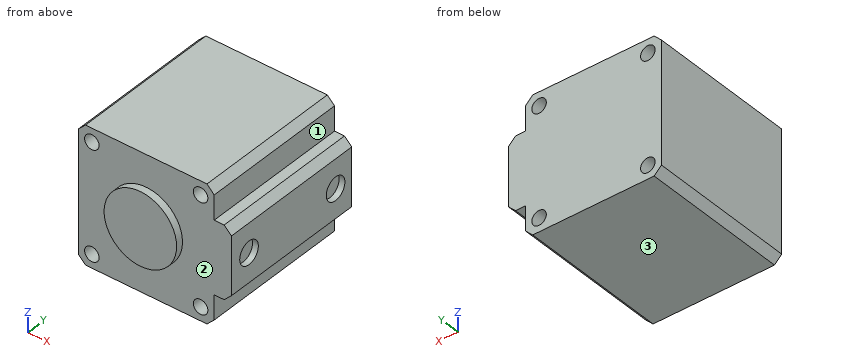
Autodesk Inventor part; units mm, degrees
ref_plane "YZ Plane" through (0, 0, 0) normal (1, 0, 0) x (0, 1, 0)
ref_plane "XZ Plane" through (0, 0, 0) normal (0, 1, 0) x (-1, 0, 0)
ref_plane "XY Plane" through (0, 0, 0) normal (0, 0, 1) x (1, 0, 0)
sketch "Sketch1" plane through (0, 0, 0) normal (0, 1, 0) x (-1, 0, 0)
  line L0 (0, 0) -> (75, 0)
  line L1 (75, 0) -> (75, -75)
  line L2 (75, -75) -> (0, -75)
  line L3 (0, -75) -> (0, 0)
  dimension "d0" = 75
  dimension "d1" = 75
extrude "Extrusion1" add sketch "Sketch1" along normal blind 82
sketch "Sketch2" plane through (0, 0, 0) normal (0, -1, 0) x (1, 0, 0)
  circle A0 centre (-37.5, -37.5) radius 20
  line L0 (0, -75) -> (0, 0)
  line L1 (-75, -75) -> (0, -75)
  dimension "d4" = 40
  dimension "d5" = 37.5
  dimension "d6" = 37.5
extrude "Extrusion2" add sketch "Sketch2" along normal blind 4
sketch "Sketch4" plane through (0, 0, 0) normal (0, -1, 0) x (1, 0, 0)
  circle A0 centre (-67.5, -7.5) radius 4
  circle A1 centre (-7.5, -7.5) radius 4
  circle A2 centre (-7.5, -67.5) radius 4
  circle A3 centre (-67.5, -67.5) radius 4
  line L0 (0, 0) -> (-75, 0)
  line L1 (0, -75) -> (0, 0)
  dimension "d12" = 8
  dimension "d13" = 8
  dimension "d14" = 8
  dimension "d15" = 8
  dimension "d16" = 60
  dimension "d17" = 60
  dimension "d18" = 60
  dimension "d19" = 60
  dimension "d20" = 60
  dimension "d21" = 60
  dimension "d22" = 7.5
  dimension "d23" = 7.5
extrude "Extrusion4" cut sketch "Sketch4" against normal blind 120.8875
sketch "Sketch5" plane through (0, 0, 0) normal (1, 0, 0) x (0, 0, -1)
  line L0 (75, 0) -> (0, 0)
  line L1 (75, 82) -> (0, 82)
  line L2 (17.5, 0) -> (57.5, 0)
  line L3 (57.5, 0) -> (57.5, 82)
  line L4 (57.5, 82) -> (17.5, 82)
  line L5 (17.5, 82) -> (17.5, 0)
  line L6 (0, 0) -> (0, 82)
  dimension "d26" = 40
  dimension "d27" = 17.5
extrude "Extrusion5" add sketch "Sketch5" along normal blind 9.5 contours L0 L5 L1 L3
sketch "Sketch6" plane through (9.5, 0, 0) normal (1, 0, 0) x (0, 0, -1)
  circle A0 centre (37.5, 12) radius 6.35
  circle A1 centre (37.5, 71) radius 6.35
  line L0 (57.5, 82) -> (17.5, 82)
  line L1 (75, 0) -> (57.5, 0)
  line L2 (75, 82) -> (0, 82)
  line L3 (37.5, 82) -> (37.5, 0)
  line L4 (0, 0) -> (75, 0)
  dimension "d30" = 12.7
  dimension "d31" = 12.7
  dimension "d32" = 11
  dimension "d33" = 12
extrude "Extrusion6" cut sketch "Sketch6" against normal blind 3.2
chamfer "Chamfer1" distance 4 angle 45 4 edges at (0, 41, -75) (-75, 41, -75) (0, 41, 0) (-75, 41, 0)
chamfer "Chamfer2" distance 4 angle 45 2 edges at (9.5, 41, -17.5) (9.5, 41, -57.5)
properties part number "SDA 63 50" material "Aluminum 6061"
Geometry: final body of the model. Coordinates: model frame, mm. Face numbers are marked on the shaded views. A direction names the side the tool comes from. Round coordinates to 2 decimals unless told otherwise and drop trailing zeros. Order: outer loops, then holes, each group sorted by start corner. A loop starts at its lowest first (then second) coordinate and runs counter-clockwise, first axis right, second up. Notation, with made-up numbers: (2, -0.5) -> (46, -0.5) arc R33 ccw to (46, 34.5) -> close; hole circle Ø2 at (82, -34). An arc over 180 degrees is marked (long way). Use one line per item in the form item = value.
(1) Section C-C on y = 25. Return loops of the section in (x, z).
Results list:
outline = (-75, -71) -> (-71, -75) -> (-4, -75) -> (0, -71) -> (0, -57.5) -> (5.5, -57.5) -> (9.5, -53.5) -> (9.5, -21.5) -> (5.5, -17.5) -> (0, -17.5) -> (0, -4) -> (-4, 0) -> (-71, 0) -> (-75, -4) -> close; hole circle Ø8 at (-67.5, -67.5); hole circle Ø8 at (-67.5, -7.5); hole circle Ø8 at (-7.5, -67.5); hole circle Ø8 at (-7.5, -7.5)
(2) Section D-D on x = -37.5. Return loops of the section in (y, z), and give its area (3 significant figures).
Results list:
outline = (-4, -57.5) -> (0, -57.5) -> (0, -75) -> (82, -75) -> (82, 0) -> (0, 0) -> (0, -17.5) -> (-4, -17.5) -> close
area = 6,310 mm^2
(3) Section B-B on z = -7.5. Return loops of the section in (x, y).
Results list:
outline = (-75, 0) -> (-71.5, 0) -> (-71.5, 82) -> (-75, 82) -> close; (-63.5, 0) -> (-11.5, 0) -> (-11.5, 82) -> (-63.5, 82) -> close; (-3.5, 0) -> (0, 0) -> (0, 82) -> (-3.5, 82) -> close
(4) Access query for the marked faces 1, 2 and 3. Directions: +Z, -Z, +X, -X, +Y, -Y. A direction counts if a zero-diameter tool reaches every point of the face in a straight line with its end or side. Return the directions, or none.
Results list:
face_1 = +Z, +X, +Y, -Y
face_2 = -Y
face_3 = -Z, +X, -X, +Y, -Y
(5) Section A-A on x = -7.5. Return loops of the section in (y, z), and give its area (3 significant figures).
Results list:
outline = (0, -75) -> (82, -75) -> (82, -71.5) -> (0, -71.5) -> close; (0, -63.5) -> (82, -63.5) -> (82, -11.5) -> (0, -11.5) -> close; (0, -3.5) -> (82, -3.5) -> (82, 0) -> (0, 0) -> close
area = 4,840 mm^2
(6) First-contact query: pin 1 Ø13 at (x, z) = (-67.5, -67.5) entering from -Y; pin 2 Ø6.5 at (y, z) = (70.5, -37.5) entering from +X; pin 3 Ø2 at (y, z) = (67.5, -19) entering from +X. Flat tips, straight axial feed; report the tip coordinate or a pass-through.
Results list:
pin_1 = 0
pin_2 = 6.3
pin_3 = 8
(7) Ray query, probe 1 along Z at (x, y) = (-67.5, 40); probe 2 along Y at (x, z) = (6.95, -37.5); probe 3 along X at (y, z) = (5, -65). Return the intervals inside material, ascending. Write a range as [from, to].
Results list:
probe_1 = [-75, -71.5], [-63.5, -11.5], [-3.5, 0]
probe_2 = [0, 5.65], [18.35, 64.65], [77.35, 82]
probe_3 = [-75, -70.62], [-64.38, -10.62], [-4.38, 0]
